```python
from build123d import *

# Parameters (mm, degrees)
F1_DEPTH = 30
F2_T     = -4
F3_W     = 4
F3_H     = 9.103521
F3_W_2   = 14.7409252822
F3_H_2   = 4.4924728572
F3_W_3   = 15.1106659323
F3_H_3   = 5.4243393242
F4_DEPTH = 26


with BuildPart() as f1:
    # F0 (on Front) → F1 (new body)
    with BuildSketch(Plane.XZ):
        Polygon((61.220897, -65.393597), (9.48831, 65.393596), (-9.284015, 65.393596), (-61.220897, -65.393597), (-41.082074, -65.393597), (-27.221939, -28.472164), (26.799398, -28.472164), (40.987162, -65.393597), align=None)
        Polygon((20.12642, -11.368643), (-20.548961, -11.368643), (-0.001722, 41.825181), align=None, mode=Mode.SUBTRACT)
    extrude(amount=F1_DEPTH)

    # F2
    f2_openings = [f1.faces().sort_by_distance(p)[0] for p in [
        (35.565629, 0, -46.290248),
    ]]
    offset(amount=F2_T, openings=f2_openings, kind=Kind.INTERSECTION)

    # F3 (on face) → F4 (join)
    with BuildSketch(Plane(origin=(0, -26, 0), x_dir=(-1, 0, 0), z_dir=(0, 1, 0))):
        Polygon((-21.9167752835, -15.368643), (-25.9167752835, -15.368643), (-29.5474826178, -24.472164), (-25.5474826178, -24.472164), align=None)
        with Locations((0, -19.9204035)):
            Rectangle(F3_W, F3_H)
        with Locations((-40.1606727391, -36.4461746067)):
            Rectangle(F3_W_2, F3_H_2)
        with Locations((-18.0124370381, 19.4464679807)):
            Rectangle(F3_W_3, F3_H_3)
        Polygon((-5.2106779282, 62.6473037582), (-8.3272252852, 60.1398882418), (-1.5950480919, 51.7722487735), (0, 49.7897122204), (1.5950480919, 51.7722487735), (8.3272252852, 60.1398882418), (5.2106779282, 62.6473037582), (0, 56.1707846416), align=None)
        with Locations((18.0124370381, 19.4464679807)):
            Rectangle(F3_W_3, F3_H_3)
        with Locations((40.1606727391, -36.4461746067)):
            Rectangle(F3_W_2, F3_H_2)
        Polygon((25.5474826178, -24.472164), (29.5474826178, -24.472164), (25.9167752835, -15.368643), (21.9167752835, -15.368643), align=None)
    extrude(amount=F4_DEPTH)


solid = f1.part
```
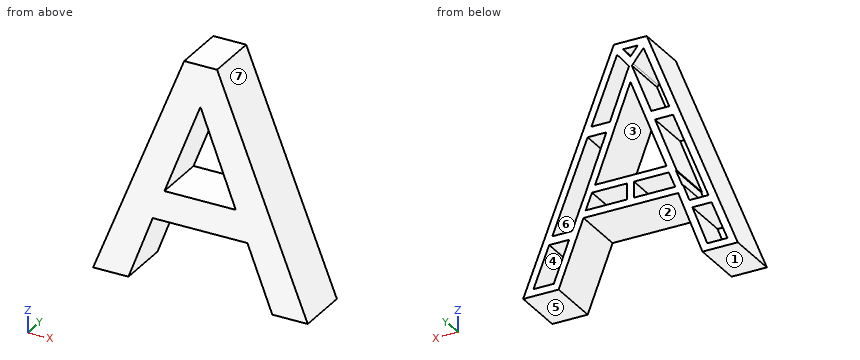
Here's how the part is built. I have some questions about the finished solid (model axes, mm). Face numbers are marked on the shaded views. A direction names the side the tool comes from. Give positions to 0.01 mm unless a question says otherwise; leave off trailing zeros. Write each loop counter-clockwise with the first axis right and the second up, starting at its lowest first coordinate (ties: lowest second). Pieces come first, ordered by that corner, then holes.
(1) Will these pins go through, and if not, where does the flat tip stop? pin 1 (2.5 mm diameter, centred on y = -11, z = -18.5, fed in from +X); pin 2 (12 mm diameter, centred on x = 21.5, z = -45.5, fed in from -Y); pin 3 (11.5 mm diameter, centred on x = 18, y = -8, fed in from -Z); pin 4 (8 mm diameter, centred on y = -15.5, z = 16, fed in from -X).
Output values:
pin 1: stops at x = 43.17
pin 2: passes through
pin 3: stops at z = -28.47
pin 4: stops at x = -30.49
(2) Imagine slicing it at B-B, the plane z = 1.5. Write out the boundary of the cut face in (x, y).
Output values:
outline: (-34.66, -30) - (-15.58, -30) - (-15.58, 0) - (-19.87, 0) - (-19.87, -26) - (-30.35, -26) - (-30.35, 0) - (-34.66, 0) - close; (15.26, -30) - (34.76, -30) - (34.76, 0) - (30.46, 0) - (30.46, -26) - (19.53, -26) - (19.53, 0) - (15.26, 0) - close
(3) Imagine slicing it at C-C, the plane x = 52.5. Write out the boundary of the cut face in (y, z), and give its area (3 significant figures).
Output values:
outline: (-30, -65.39) - (0, -65.39) - (0, -61.39) - (-26, -61.39) - (-26, -54.22) - (0, -54.22) - (0, -43.35) - (-30, -43.35) - close
area: 475 mm2
(4) If I drill on L1, parallel to X at y = -15.5, z = 7.5; L2, parallel to X at y = -19.75, z = -50; L3, parallel to X at y = -11.75, z = -19, over which ranges is the centre line in solid material (lowest first)?
Output values:
L1: x = -32.27 to -27.97, -17.55 to -13.26, 12.99 to 17.26, 28.09 to 32.39
L2: x = -55.11 to -50.8, -39.58 to -35.3, 35.07 to 39.36, 50.83 to 55.13
L3: x = -42.8 to -38.49, -27.37 to -23.37, -2 to 2, 23.37 to 27.37, 38.57 to 42.87
(5) Thinking about a two-plate mould opening in Z: for the marked faces 4, 5, 6 and 7, which applies, pulls with the +Z half, pulls with the -Z half, needs draft (parallel to the pull), parting line crosses it, or undercut?
Output values:
face 4: undercut
face 5: pulls with the -Z half
face 6: undercut
face 7: pulls with the +Z half
(6) Imagine slicing it at D-D, the plane z = -50. Write out the boundary of the cut face in (x, y), and give its area (3 significant figures).
Output values:
outline: (-55.11, -30) - (-35.3, -30) - (-35.3, 0) - (-39.58, 0) - (-39.58, -26) - (-50.8, -26) - (-50.8, 0) - (-55.11, 0) - close; (35.07, -30) - (55.13, -30) - (55.13, 0) - (50.83, 0) - (50.83, -26) - (39.36, -26) - (39.36, 0) - (35.07, 0) - close
area: 606 mm2
(7) On a 3-axis mill with a long thin cutter (end or side, diameter ignored), from which of +Z, -Z, +X, -X, +Y, -Y can I reach the whole of each face in a straight line? I mean the marked faces 1, 2 and 3. Say none if no direction works.
Output values:
face 1: -Z, +X, -X, +Y, -Y
face 2: -Z, +Y, -Y
face 3: +Y, -Y
(8) Imagine slicing it at A-A, the plane y = -27.5. Write out the boundary of the cut face in (x, z), and give its area (3 significant figures).
Output values:
outline: (-61.22, -65.39) - (-41.08, -65.39) - (-27.22, -28.47) - (26.8, -28.47) - (40.99, -65.39) - (61.22, -65.39) - (9.49, 65.39) - (-9.28, 65.39) - close; hole (-20.55, -11.37) - (20.13, -11.37) - (0, 41.83) - close
area: 5,640 mm2
